```python
from build123d import *

# Parameters (mm, degrees)
SKETCH1_W           = 16
SKETCH1_H           = 16
BOSS_EXTRUDE1_DEPTH = 10
SKETCH2_R           = 2
BOSS_EXTRUDE2_DEPTH = 2
SHELL1_T            = -1
SKETCH3_R           = 2.7
SKETCH3_R_2         = 1.7
BOSS_EXTRUDE3_DEPTH = 9


with BuildPart() as part:
    # Sketch1 → Boss-Extrude1 (new body)
    with BuildSketch(Plane(origin=(0, 0, 0), x_dir=(1, 0, 0), z_dir=(0, 1, 0))):
        Rectangle(SKETCH1_W, SKETCH1_H)
    extrude(amount=BOSS_EXTRUDE1_DEPTH)

    # Sketch2 → Boss-Extrude2 (add)
    with BuildSketch(Plane(origin=(0, 10, 0), x_dir=(1, 0, 0), z_dir=(0, 1, 0))):
        with Locations((-4, 4)):
            Circle(SKETCH2_R)
        with Locations((4, 4)):
            Circle(SKETCH2_R)
        with Locations((-4, -4)):
            Circle(SKETCH2_R)
        with Locations((4, -4)):
            Circle(SKETCH2_R)
    extrude(amount=BOSS_EXTRUDE2_DEPTH)

    # Shell1
    shell1_openings = [part.faces().sort_by_distance(p)[0] for p in [
        (0, 0, 0),
    ]]
    offset(amount=SHELL1_T, openings=shell1_openings, kind=Kind.INTERSECTION)

    # Sketch3 → Boss-Extrude3 (add)
    with BuildSketch(Plane.XZ.offset(-9)):
        Circle(SKETCH3_R)
        Circle(SKETCH3_R_2, mode=Mode.SUBTRACT)
    extrude(amount=BOSS_EXTRUDE3_DEPTH)


solid = part.part
```
Model file for the job. Use its own axes, mm. A direction names the side the tool comes from. Coordinates: 2 decimals unless noted, no trailing zeros. Loops run counter-clockwise (first coordinate to the right, second up) from the corner with the lowest first, then second, coordinate; pieces in that order, holes last. Notation, with made-up numbers: (56, 56) - (107, 56) arc R30 cw to (107, 81) - close; hole circle Ø5 at (-6, 3). An arc over 180 degrees is marked (long way). Write item = value, one per line. Start each with the question number.
Item 1: Saw through at A-A, the plane y = 3.5. List the corners of the cut face in (x, z), then the cut area to 3 significant figures.
Item 2: Saw through at D-D, the plane y = 9.5. List the corners of the cut face in (x, z).
Item 3: Saw through at C-C, the plane z = -4. List the corners of the cut face in (x, y), then the cut area to 3 significant figures.
Item 4: Pull direction X, two halves, no side cores. Call faces 4 (the face through (-5.6, 11, -2.8)), 5 (the face through (-8, 5, 0)), 6 (the face through (-3, 9, 0)), 7 (the face through (4, 12, -4)): +X half, -X half, draft (parallel to the pull), parting line (faces both ways), or undercut.
Item 5: Wall check: probe 1 along Z at (x, y) = (-4, 10.05); probe 2 along Z at (x, y) = (-2.75, 4.25). Give the ranges that are in metal, low to high. Write a range as [from, to].
Item 6: Drop flat-ended pins along their axis: pin 1 Ø1.6 at (x, z) = (3.5, 4) entering from -Y; pin 2 Ø1.6 at (x, z) = (4, -4) entering from -Y; pin 3 Ø3 at (x, z) = (-1.5, 0.5) entering from +Y. Give the stop position or say it passes through.
Item 7: Saw through at B-B, the plane x = 6.25. List the corners of the cut face in (y, z), then the cut area to 3 significant figures.
Item 8: 3-axis set-ups, long thin cutter, end or side, ignore diameter. For faces 1 (the face through (0, 10, 0)), 2 (the face through (-4, 11, 4)), 3 (the face through (4, 12, 4)): which of +Z, -Z, +X, -X, +Y, -Y reach the whole face in a straight line?
Answers:
q1.outline = (-8, -8) - (8, -8) - (8, 8) - (-8, 8) - close; circle Ø5.4 at (0, 0); hole (-7, -7) - (7, -7) - (7, 7) - (-7, 7) - close; hole circle Ø3.4 at (0, 0)
q1.area = 73.8 mm2
q2.outline = (-8, -8) - (8, -8) - (8, 8) - (-8, 8) - close; hole circle Ø2 at (-4, -4); hole circle Ø2 at (-4, 4); hole circle Ø2 at (4, -4); hole circle Ø2 at (4, 4)
q3.outline = (-8, 0) - (-7, 0) - (-7, 9) - (-5, 9) - (-5, 11) - (-3, 11) - (-3, 9) - (3, 9) - (3, 11) - (5, 11) - (5, 9) - (7, 9) - (7, 0) - (8, 0) - (8, 10) - (6, 10) - (6, 12) - (2, 12) - (2, 10) - (-2, 10) - (-2, 12) - (-6, 12) - (-6, 10) - (-8, 10) - close
q3.area = 42.0 mm2
q4.face_4 = undercut
q4.face_5 = -X half
q4.face_6 = undercut
q4.face_7 = draft
q5.probe_1 = [-6, -5], [-3, -2], [2, 3], [5, 6]
q5.probe_2 = [-8, -7], [7, 8]
q6.pin_1 = 9
q6.pin_2 = 11
q6.pin_3 = 10
q7.outline = (0, -8) - (10, -8) - (10, 8) - (0, 8) - (0, 7) - (9, 7) - (9, -7) - (0, -7) - close
q7.area = 34.0 mm2
q8.face_1 = +Y
q8.face_2 = -Y
q8.face_3 = +Z, -Z, +X, -X, +Y
